from build123d import *

# Parameters (mm, degrees)
ESQUISSE1_W             = 21
ESQUISSE1_H             = 100
BOSS_EXTRU_1_DEPTH      = 10
ESQUISSE2_R             = 2
ESQUISSE2_R_2           = 2.5
ENL_V_MAT_EXTRU_1_DEPTH = 10
CONG_1_R                = 5
ENL_V_MAT_EXTRU_2_DEPTH = 4
ESQUISSE4_R             = 3.75
ENL_V_MAT_EXTRU_4_DEPTH = 4


with BuildPart() as part:
    # Esquisse1 → Boss.-Extru.1 (new body)
    with BuildSketch(Plane.XY):
        with Locations((2.217198679, -40)):
            Rectangle(ESQUISSE1_W, ESQUISSE1_H)
    extrude(amount=BOSS_EXTRU_1_DEPTH)

    # Esquisse2 → Enlèv. mat.-Extru.1 (cut)
    with BuildSketch(Plane.XY.offset(10)):
        with Locations((2.217198679, 0)):
            Circle(ESQUISSE2_R)
        with Locations((2.217198679, -25)):
            Circle(ESQUISSE2_R)
        with Locations((2.217198679, -80)):
            Circle(ESQUISSE2_R_2)
    extrude(amount=-ENL_V_MAT_EXTRU_1_DEPTH, mode=Mode.SUBTRACT)

    # Congé1
    cong_1_edges = [part.edges().sort_by_distance(p)[0] for p in [
        (-8.282801321, 10, 5),
        (12.717198679, 10, 5),
        (12.717198679, -90, 5),
        (-8.282801321, -90, 5),
    ]]
    fillet(cong_1_edges, radius=CONG_1_R)

    # Esquisse3 → Enlèv. mat.-Extru.2 (cut)
    with BuildSketch(Plane(origin=(0, 0, 0), x_dir=(-1, 0, 0), z_dir=(0, 0, -1))):
        Polygon((-3.80491192, 2.75), (-5.39262516, 0), (-3.80491192, -2.75), (-0.629485439, -2.75), (0.958227801, 0), (-0.629485439, 2.75), align=None)
        Polygon((-3.80491192, -22.25), (-5.39262516, -25), (-3.80491192, -27.75), (-0.629485439, -27.75), (0.958227801, -25), (-0.629485439, -22.25), align=None)
    extrude(amount=-ENL_V_MAT_EXTRU_2_DEPTH, mode=Mode.SUBTRACT)

    # Esquisse4 → Enlèv. mat.-Extru.4 (cut)
    with BuildSketch(Plane.XY.offset(10)):
        with Locations((2.217198679, -80)):
            Circle(ESQUISSE4_R)
    extrude(amount=-ENL_V_MAT_EXTRU_4_DEPTH, mode=Mode.SUBTRACT)


solid = part.part
Can you work these out from the model? Positions are in its coordinate system, mm. A direction names the side the tool comes from. Give positions to 0.01 mm unless a question says otherwise; leave off trailing zeros. Loops run counter-clockwise (first coordinate to the right, second up) from the corner with the lowest first, then second, coordinate; pieces in that order, holes last. Notation, with made-up numbers: (-11, 87.25) -> (-6, 87.25) arc R34 ccw to (-6, 120.25) -> close; hole circle Ø4 at (10.25, 47.25). An arc over 180 degrees is marked (long way). Return JSON: item names as keys, results as strings.
Q1. On a 3-axis mill with a long thin cutter (end or side, diameter ignored), from which of +Z, -Z, +X, -X, +Y, -Y can I reach the whole of each face in a straight line? I mean faces 4 (the face through (-0.153, -26.394, 1.972)), 5 (the face through (11.214, -88.574, 5.07)). Say none if no direction works.
Checks:
{"face 4": "-Z", "face 5": "+Z, -Z, +X, -Y"}
Q2. I want a section at B-B, the plane z = 1.5. List the corners of the cut face in (x, y) for me.
Checks:
{"outline": "(-8.28, -85) arc R5 ccw to (-3.28, -90) -> (7.72, -90) arc R5 ccw to (12.72, -85) -> (12.72, 5) arc R5 ccw to (7.72, 10) -> (-3.28, 10) arc R5 ccw to (-8.28, 5) -> close; hole (-0.96, -25) -> (0.63, -27.75) -> (3.8, -27.75) -> (5.39, -25) -> (3.8, -22.25) -> (0.63, -22.25) -> close; hole (-0.96, 0) -> (0.63, -2.75) -> (3.8, -2.75) -> (5.39, 0) -> (3.8, 2.75) -> (0.63, 2.75) -> close; hole circle Ø5 at (2.22, -80)"}
Q3. I want a section at A-A, the plane y = -80. List the corners of the cut face in (x, z) for me, then the cut area to 3 significant figures.
Checks:
{"outline": "(-8.28, 0) -> (-0.28, 0) -> (-0.28, 6) -> (-1.53, 6) -> (-1.53, 10) -> (-8.28, 10) -> close; (4.72, 0) -> (12.72, 0) -> (12.72, 10) -> (5.97, 10) -> (5.97, 6) -> (4.72, 6) -> close", "area": "150 mm2"}
Q4. For pin 1 Ø3 at (x, z) = (-5.5, 5.5) entering from +Y; pin 2 Ø3 at (x, y) = (2.22, -25) entering from -Z; pin 3 Ø4.5 at (x, y) = (2.22, 0) entering from -Z, each with a flat end and sliding along its axis, tell me the tip position at first contact or that it passes through.
Checks:
{"pin 1": "stops at y = 9.95", "pin 2": "passes through", "pin 3": "stops at z = 4"}
Q5. We'd pull the mould along Y, two halves only. Please class faces 1 (the face through (11.214, 8.574, 5.07)), 2 (the face through (2, -39, 0)), 3 (the face through (2, 2.75, 2)): released by +Y, released by -Y, zero draft, split by the parting line, or undercut.
Checks:
{"face 1": "released by +Y", "face 2": "zero draft", "face 3": "undercut"}
Q6. I need wall thicknesses on probe 1 along Y at (x, z) = (1.5, 1.5); probe 2 along Y at (x, z) = (1.75, 3); probe 3 along Y at (x, z) = (-0.5, 8.25). Which ranges of each line are inside material? Lowest first, please.
Checks:
{"probe 1": "y = -90 to -82.39, -77.61 to -27.75, -22.25 to -2.75, 2.75 to 10", "probe 2": "y = -90 to -82.46, -77.54 to -27.75, -22.25 to -2.75, 2.75 to 10", "probe 3": "y = -90 to -82.58, -77.42 to 10"}
